```python
from build123d import *

# Parameters (mm, degrees)
F0_R     = 50.8
F0_R_2   = 7.14375
F1_DEPTH = 6.35
F2_W     = 25.4
F2_H     = 25.4
F3_DEPTH = 127
F4_R     = 6.35
F5_DEPTH = 1041.4
F6_W     = 25.4
F6_H     = 25.4
F7_DEPTH = 127


with BuildPart() as f1:
    # F0 (on Front) → F1 (new body)
    with BuildSketch(Plane.XZ):
        Circle(F0_R)
        with Locations((-11.773547, -36.235253)):
            Circle(F0_R_2, mode=Mode.SUBTRACT)
        with Locations((-30.823547, -22.394618)):
            Circle(F0_R_2, mode=Mode.SUBTRACT)
        with Locations((-38.1, 0)):
            Circle(F0_R_2, mode=Mode.SUBTRACT)
        with Locations((11.773547, -36.235253)):
            Circle(F0_R_2, mode=Mode.SUBTRACT)
        with Locations((30.823547, -22.394618)):
            Circle(F0_R_2, mode=Mode.SUBTRACT)
        with Locations((38.1, 0)):
            Circle(F0_R_2, mode=Mode.SUBTRACT)
        with Locations((-30.823547, 22.394618)):
            Circle(F0_R_2, mode=Mode.SUBTRACT)
        with Locations((-11.773547, 36.235253)):
            Circle(F0_R_2, mode=Mode.SUBTRACT)
        with Locations((30.823547, 22.394618)):
            Circle(F0_R_2, mode=Mode.SUBTRACT)
        with Locations((11.773547, 36.235253)):
            Circle(F0_R_2, mode=Mode.SUBTRACT)
    extrude(amount=F1_DEPTH)



with BuildPart() as f3:
    # F2 (on face) → F3 (new body)
    with BuildSketch(Plane(origin=(0, 1041.4, 0), x_dir=(-1, 0, 0), z_dir=(0, 1, 0))):
        Rectangle(F2_W, F2_H)
    extrude(amount=F3_DEPTH)


with BuildPart() as f1_1:
    add(f1.part)

    add(f3.part)  # F5 merges F3
    # F4 (on face) → F5 (join)
    with BuildSketch(Plane(origin=(0, 0, 0), x_dir=(-1, 0, 0), z_dir=(0, 1, 0))):
        Circle(F4_R)
    extrude(amount=F5_DEPTH)

    # F6 (on face) → F7 (join)
    with BuildSketch(Plane.XZ.offset(6.35)):
        Rectangle(F6_W, F6_H)
    extrude(amount=F7_DEPTH)


solid = f1_1.part
```
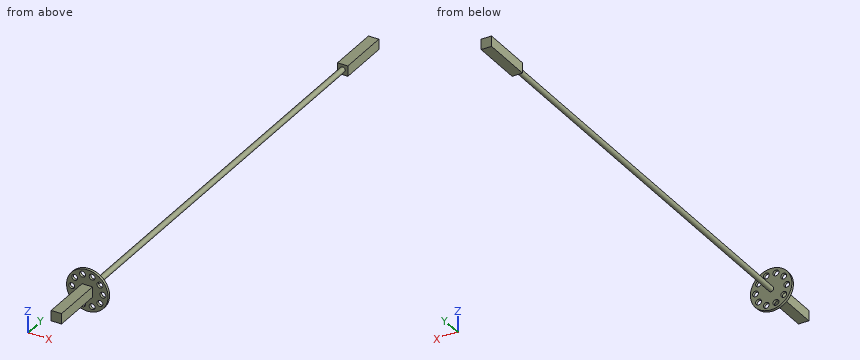
Can you work these out from the model? Positions are in its coordinate system, mm. Coordinates: 2 decimals unless noted, no trailing zeros. Loops run counter-clockwise (first coordinate to the right, second up) from the corner with the lowest first, then second, coordinate; pieces in that order, holes last. Notation, with made-up numbers: (71, -16) -> (87, -16) arc R13 ccw to (87, -2) -> close; hole circle Ø8 at (9, -17.5). An arc over 180 degrees is marked (long way). Put each result on its own line as item: value. Start each with the question number.
Q1. I want a section at A-A (y = 621.5). Write out the boundary of the cut face in (x, z).
Q2. I'm going to push flat-ended pins straight in: P1, Ø12, axis at x = -5, z = 29.5, coming from the -Y side; P2, Ø18.5, axis at x = -30.82, z = -22.39, coming from the +Y side; P3, Ø12.5, axis at y = -53.5, z = -6, coming from the -X side. Where does each tip first touch, or does it pass through?
Q3. If I drill on line 1 (Y direction, x = 10.5, z = -11); line 2 (Y direction, x = 44, z = -9); line 3 (Z direction, x = -38.1, y = -4), over which ranges is the centre line in solid material (lowest first)? Write a range as [from, to].
Taken from the geometry:
1. outline: circle Ø12.7 at (0, 0)
2. P1: stops at y = -6.35
2. P2: stops at y = 0
2. P3: stops at x = -12.7
3. line 1: y = [-133.35, 0], [1041.4, 1168.4]
3. line 2: y = [-6.35, 0]
3. line 3: z = [-33.6, -7.14], [7.14, 33.6]
